Here's how the part is built. I have some questions about the finished solid (model axes, mm). A direction names the side the tool comes from. Coordinates: 2 decimals unless noted, no trailing zeros. Loops run counter-clockwise (first coordinate to the right, second up) from the corner with the lowest first, then second, coordinate; pieces in that order, holes last. Notation, with made-up numbers: M -13,-25 L 6,-25 A12 ccw 6,-17 Z; hole C -27,59.5 d5. An arc over 180 degrees is marked long. Use CSV: the item, a comma, the result in double quotes. Start each with the question number.
Q1. Which directions (+Z, -Z, +X, -X, +Y, -Y) give clear straight access to the entire face, cutting with the end or side of a thin tool? Please do faces 4 (the flat face through (-10, 6, 30)), 5 (the flat face through (-160, 0, 0)).
Q2. Please list where these lines run through material, in increasing order: probe 1 along Y at (x, z) = (-102, -10.5); probe 2 along X at (y, z) = (30, -16.5). Write a range as [from, to].
Q3. If we section it at C-C (x = -29.5): Please give me the cut outline in (y, z).
Q4. If we section it at A-A (z = 0): Please give me the cut outline in (x, y).
Q5. For pin 1 Ø2 at (x, z) = (-114, 10) entering from -Y; pin 2 Ø8 at (x, y) = (-116.5, -16.5) entering from +Z; pin 3 Ø10 at (y, z) = (-1.5, 7.5) entering from -X; pin 4 Ø2 at (x, z) = (-83, 2.5) entering from +Y, each with a flat end and sliding along its axis, tell me the tip position at first contact or that it passes through.
Q6. If we section it at D-D (x = -141.5): Please give me the cut outline in (y, z).
Q7. If we mould it in two halves opening along X, with no side actions, what happens to faces 1 (the flat face through (0, 0, 0)), 2 (the cylindrical face through (-76.784, -4.336, 19.524)), 3 (the flat face through (-135, 7, -4))? For each: +X half, -X half, draft (parallel to the pull), parting line (faces both ways), or undercut.
Autodesk Inventor part; units mm, degrees
ref_plane "YZ Plane" through (0, 0, 0) normal (1, 0, 0) x (0, 1, 0)
ref_plane "XZ Plane" through (0, 0, 0) normal (0, 1, 0) x (-1, 0, 0)
ref_plane "XY Plane" through (0, 0, 0) normal (0, 0, 1) x (1, 0, 0)
sketch "草圖1" plane through (0, 0, 0) normal (0, 0, 1) x (1, 0, 0)
  line L0 (0, 0) -> (0, 30)
  line L1 (-10, 30) -> (-20, 20)
  line L2 (-20, 20) -> (-132, 20)
  line L3 (-132, 20) -> (-135, 17)
  line L4 (-135, 17) -> (-135, 7.5)
  line L5 (-135, 7.5) -> (-160, 7.5)
  line L6 (-160, 7.5) -> (-160, 0)
  line L7 (-160, 0) -> (0, 0)
  line L8 (-10, 30) -> (-10, 40)
  line L9 (-10, 40) -> (0, 30)
  dimension "d3" = 45
  dimension "d4" = 150
  dimension "d5" = 7.5
  dimension "d6" = 25
  dimension "d7" = 45
  dimension "d8" = 3
  dimension "d9" = 20
  dimension "d10" = 160
  dimension "d11" = 40
  dimension "d12" = 10
revolve "迴轉1" add sketch "草圖1" angle 360 about axis through (-160, 0, 0) along (1, 0, 0)
properties part number "2-2-2"
Results below:
1,face 4,"-X"
1,face 5,"+Z, -Z, -X, +Y, -Y"
2,probe 1,"[-17.02, 17.02]"
2,probe 2,"[-10, -4.24]"
3,outline,"C 0,0 d40"
4,outline,"M -160,-7.5 L -135,-7.5 L -135,-17 L -132,-20 L -20,-20 L -10,-30 L -10,-40 L 0,-30 L 0,30 L -10,40 L -10,30 L -20,20 L -132,20 L -135,17 L -135,7.5 L -160,7.5 Z"
5,pin 1,"y = -17.86"
5,pin 2,"z = 15.61"
5,pin 3,"x = -160"
5,pin 4,"y = 19.94"
6,outline,"C 0,0 d15"
7,face 1,"+X half"
7,face 2,"draft"
7,face 3,"-X half"
